Read the model definition and answer for the solid it produces. Units are mm, in the model's axes. A direction names the side the tool comes from. Coordinates: 2 decimals unless noted, no trailing zeros. Order: outer loops, then holes, each group sorted by start corner. A loop starts at its lowest first (then second) coordinate and runs counter-clockwise, first axis right, second up. Notation, with made-up numbers: (48.25, 1.25) - (60.25, 1.25) arc R27 cw to (60.25, 26.25) - close; hole circle Ø9 at (42, 69). An arc over 180 degrees is marked (long way). Use one line per item in the form item = value.
```python
from build123d import *

# Parameters (mm, degrees)
BOSS_EXTRUDE3_DEPTH     = 70
FILLET7_R               = 5
FILLET8_R               = 5
FILLET9_R               = 5
FILLET10_R              = 5
ESQUISSE3_W             = 30
ESQUISSE3_H             = 60
ENL_V_MAT_EXTRU_1_DEPTH = 107.418983269
ESQUISSE5_W             = 10
ESQUISSE5_H             = 60
ENL_V_MAT_EXTRU_2_DEPTH = 107.418983269
ESQUISSE13_R            = 0.75
ENL_V_MAT_EXTRU_3_DEPTH = 10
ESQUISSE4_R             = 0.75
ENL_V_MAT_EXTRU_6_DEPTH = 10


with BuildPart() as part:
    # Sketch1 → Boss-Extrude3 (new body)
    with BuildSketch(Plane(origin=(0, 0, 0), x_dir=(1, 0, 0), z_dir=(0, 1, 0))):
        Polygon((-75, 0), (-75, 10), (25, 10), (1.715728753, 33.284271247), (1.715728753, 38.284271247), (30, 10), (58.284271247, 38.284271247), (58.284271247, 33.284271247), (35, 10), (25, 0), align=None)
    extrude(amount=BOSS_EXTRUDE3_DEPTH)

    # Fillet7
    fillet7_edges = [part.edges().sort_by_distance(p)[0] for p in [
        (30, 35, -10),
    ]]
    fillet(fillet7_edges, radius=FILLET7_R)

    # Fillet8
    fillet8_edges = [part.edges().sort_by_distance(p)[0] for p in [
        (25, 35, -10),
    ]]
    fillet(fillet8_edges, radius=FILLET8_R)

    # Fillet9
    fillet9_edges = [part.edges().sort_by_distance(p)[0] for p in [
        (58.284271247, 35, -33.284271247),
        (1.715728753, 35, -33.284271247),
    ]]
    fillet(fillet9_edges, radius=FILLET9_R)

    # Fillet10
    fillet10_edges = [part.edges().sort_by_distance(p)[0] for p in [
        (25, 35, 0),
    ]]
    fillet(fillet10_edges, radius=FILLET10_R)

    # Esquisse3 → Enlèv. mat.-Extru.1 (cut, through all)
    with BuildSketch(Plane(origin=(0, 0, -10), x_dir=(-1, 0, 0), z_dir=(0, 0, -1))):
        with Locations((60, 35)):
            Rectangle(ESQUISSE3_W, ESQUISSE3_H)
    extrude(amount=-ENL_V_MAT_EXTRU_1_DEPTH, mode=Mode.SUBTRACT)

    # Esquisse5 → Enlèv. mat.-Extru.2 (cut, through all)
    with BuildSketch(Plane(origin=(0, 0, -10), x_dir=(-1, 0, 0), z_dir=(0, 0, -1))):
        with Locations((40, 35)):
            Rectangle(ESQUISSE5_W, ESQUISSE5_H)
    extrude(amount=-ENL_V_MAT_EXTRU_2_DEPTH, mode=Mode.SUBTRACT)

    # Esquisse13 → Enlèv. mat.-Extru.3 (cut)
    with BuildSketch(Plane(origin=(0, 65, 0), x_dir=(-1, 0, 0), z_dir=(0, -1, 0))):
        with Locations(Location((44, 5, 0), (0, 0, 90))):
            Circle(ESQUISSE13_R)
    extrude(amount=-ENL_V_MAT_EXTRU_3_DEPTH, mode=Mode.SUBTRACT)

    # Esquisse4 → Enlèv. mat.-Extru.6 (cut)
    with BuildSketch(Plane.XZ.offset(-65)):
        with Locations((-73, -5)):
            Circle(ESQUISSE4_R)
        with Locations((-68, -5)):
            Circle(ESQUISSE4_R)
        with Locations((-70.5, -5)):
            Circle(ESQUISSE4_R)
        with Locations((-65.5, -5)):
            Circle(ESQUISSE4_R)
        with Locations((-46.5, -5)):
            Circle(ESQUISSE4_R)
        with Locations((-49, -5)):
            Circle(ESQUISSE4_R)
        with Locations((-51.5, -5)):
            Circle(ESQUISSE4_R)
    extrude(amount=-ENL_V_MAT_EXTRU_6_DEPTH, mode=Mode.SUBTRACT)


solid = part.part
```
(1) Section A-A, the plane x = -37 is taken. Write down the section's boundary in (y, z).
Answer list:
outline = (0, -10) - (5, -10) - (5, 0) - (0, 0) - close; (65, -10) - (70, -10) - (70, 0) - (65, 0) - close
(2) Section C-C, the plane y = 62.5 is taken. Write down the section's boundary in (x, z), then the cut area to 3 significant figures.
Answer list:
outline = (-35, -10) - (12.93, -10) arc R5 cw to (16.46, -18.54) - (3.18, -31.82) arc R5 ccw to (1.72, -35.36) - (1.72, -38.28) - (26.46, -13.54) arc R5 cw to (33.54, -13.54) - (58.28, -38.28) - (58.28, -35.36) arc R5 ccw to (56.82, -31.82) - (26.46, -1.46) arc R5 ccw to (22.93, 0) - (-35, 0) - close
area = 942 mm2
(3) Section D-D, the plane x = -8.5 is taken. Write down the section's boundary in (y, z).
Answer list:
outline = (0, -10) - (70, -10) - (70, 0) - (0, 0) - close
(4) Section B-B, the plane z = -16 is taken. Write down the section's boundary in (x, y).
Answer list:
outline = (17.83, 0) - (24, 0) - (24, 70) - (17.83, 70) - close; (36, 0) - (41, 0) - (41, 70) - (36, 70) - close
(5) Which of the six approach directions +Z, -Z, +X, -X, +Y, -Y give full straight-line access (tool end or side, diameter ignored) to faces 5 (the flat face through (-55, 5, -5)), 6 (the flat face through (10, 35, -25)), 7 (the flat face through (46, 35, -26)), 8 (the cylindrical face through (57.893, 35.49, -33.417))?
Answer list:
face_5 = +Z, -Z, -X
face_6 = -X, +Y, -Y
face_7 = -Z, +Y, -Y
face_8 = +Z, +X, +Y, -Y
(6) Straight lines are drawn through the part: L1, parallel to Z at x = -44, y = 66.6; L2, parallel to Y at x = -60, z = -8; L3, parallel to Z at x = -61.5, y = 4. For each, find the intervals that lie inside material, in ascending order.
Answer list:
L1 = -10 to -5.75, -4.25 to 0
L2 = 0 to 5, 65 to 70
L3 = -10 to 0
(7) The mould has two halves that part along X. Classify faces 1 (the flat face through (58.284, 35, -37)), 2 (the cylindrical face through (29.95, 35.49, -12.07)), 3 (the flat face through (-14, 35, 0)), 4 (the flat face through (14, 35, -26)): +X half, -X half, draft (parallel to the pull), parting line (faces both ways), or undercut.
Answer list:
face_1 = +X half
face_2 = undercut
face_3 = draft
face_4 = undercut
(8) Given pin 1 Ø12 at (y, z) = (60.5, -22.5) entering from -X; pin 2 Ø3 at (y, z) = (33, -29.5) entering from -X; pin 3 Ø10 at (y, z) = (26.5, -33) entering from -X, each flat-ended and moving along its own axis, determine where each tip first touches the part or whether it passes through.
Answer list:
pin_1 = 6.5
pin_2 = 4
pin_3 = 1.72
